The listing builds one solid part. Answer for the finished solid, in the listing's coordinates (mm). A direction names the side the tool comes from. Coordinates: 2 decimals unless noted, no trailing zeros. Write each loop counter-clockwise with the first axis right and the second up, starting at its lowest first coordinate (ties: lowest second). Pieces come first, ordered by that corner, then holes.
from build123d import *

# Parameters (mm, degrees)
SKETCH2_R                = 5
SKETCH2_R_2              = 1.5
HOLES_DEPTH              = 4
SPOKES_DEPTH             = 4
FILLET2_R                = 2
CIRPATTERN2_COUNT        = 4
FILLET2_OF_CIRPATTERN2_R = 2


with BuildPart() as part:
    # Sketch1 → Revolve1 (revolve)
    with BuildSketch(Plane.XY):
        Polygon((2, 0), (2, 39), (17, 39), (17, 44), (0, 44), (0, 0), align=None)
    revolve1 = revolve(axis=Axis((2, 0, 0), (-1, 0, 0)))

    # Mirror1: Revolve1 across plane
    add(revolve1.mirror(Plane.ZY))

    # Sketch2 → holes (cut)
    with BuildSketch(Plane(origin=(2, 0, 0), x_dir=(0, 0, -1), z_dir=(1, 0, 0))):
        with Locations(Location((0, 0, 0), (0, 0, 90))):
            Circle(SKETCH2_R)
        with Locations(Location((8, 0, 0), (0, 0, 90))):
            Circle(SKETCH2_R_2)
        with Locations(Location((0, -8, 0), (0, 0, 90))):
            Circle(SKETCH2_R_2)
        with Locations(Location((-8, 0, 0), (0, 0, 90))):
            Circle(SKETCH2_R_2)
        with Locations(Location((0, 8, 0), (0, 0, 90))):
            Circle(SKETCH2_R_2)
    extrude(amount=-HOLES_DEPTH, mode=Mode.SUBTRACT)

    # Sketch3 → spokes (cut)
    with BuildSketch(Plane(origin=(2, 0, 0), x_dir=(0, 0, -1), z_dir=(1, 0, 0))):
        with BuildLine():
            Line((8.131727984, 16.131727984), (16.131727984, 8.131727984))
            Line((16.131727984, 8.131727984), (31.131727984, 8.131727984))
            ThreePointArc((31.131727984, 8.131727984), (22.752027242, 22.752027242), (8.131727984, 31.131727984))
            Line((8.131727984, 31.131727984), (8.131727984, 16.131727984))
        make_face()
    spokes = extrude(amount=-SPOKES_DEPTH, mode=Mode.SUBTRACT)

    # Fillet2
    fillet2_edges = [part.edges().sort_by_distance(p)[0] for p in [
        (0, 16.131727984, -8.131727984),
        (0, 8.131727984, -16.131727984),
        (0, 8.131727984, -31.131727984),
        (0, 31.131727984, -8.131727984),
    ]]
    fillet(fillet2_edges, radius=FILLET2_R)

    # CirPattern2: spokes ×4 about axis
    cirpattern2_axis = Axis((0, 0, 0), (1, 0, 0))
    for i in range(1, CIRPATTERN2_COUNT):
        add(spokes.rotate(cirpattern2_axis, i * 360 / CIRPATTERN2_COUNT), mode=Mode.SUBTRACT)

    # Fillet2 of CirPattern2
    fillet2_of_cirpattern2_edges = [part.edges().sort_by_distance(p)[0] for p in [
        (0, 8.131727984, 16.131727984),
        (0, 16.131727984, 8.131727984),
        (0, 31.131727984, 8.131727984),
        (0, 8.131727984, 31.131727984),
        (0, -16.131727984, 8.131727984),
        (0, -8.131727984, 16.131727984),
        (0, -8.131727984, 31.131727984),
        (0, -31.131727984, 8.131727984),
        (0, -8.131727984, -16.131727984),
        (0, -16.131727984, -8.131727984),
        (0, -31.131727984, -8.131727984),
        (0, -8.131727984, -31.131727984),
    ]]
    fillet(fillet2_of_cirpattern2_edges, radius=FILLET2_OF_CIRPATTERN2_R)


solid = part.part
1. Flat-ended cylindrical pins translate along their axes: P1, Ø1.2, axis at x = 0, z = 20, coming from the -Y side; P2, Ø12, axis at x = -1.5, y = 4.5, coming from the -Z side; P3, Ø2, axis at x = 0, y = 24.5, coming from the +Z side. Find the tip coordinate at first contact, or state that the pin passes through.
Results found:
P1: stops at y = -39.49
P2: stops at z = -44
P3: stops at z = 37.2
2. A tool of negligible diameter and unlimited length cuts with its end or side. For faces 1 (the flat face through (-2, -8, 8)), 2 (the cylindrical face through (0.028, -22.893, -22.61)), 3 (the flat face through (2, -8, 8)), from which of +Z, -Z, +X, -X, +Y, -Y can it reach the whole face along a straight path? Write none if from no direction.
Results found:
face 1: -X
face 2: +X, -X
face 3: +X
3. Section A-A on z = 0 is taken. Give the vertices of the cut face in (x, y).
Results found:
outline: (-17, -44) - (17, -44) - (17, -39) - (2, -39) - (2, -9.5) - (-2, -9.5) - (-2, -39) - (-17, -39) - close; (-17, 39) - (-2, 39) - (-2, 9.5) - (2, 9.5) - (2, 39) - (17, 39) - (17, 44) - (-17, 44) - close; (-2, -6.5) - (2, -6.5) - (2, -5) - (-2, -5) - close; (-2, 5) - (2, 5) - (2, 6.5) - (-2, 6.5) - close
4. Section B-B on x = -3.5 is taken. Give the vertices of the cut face in (y, z).
Results found:
outline: circle Ø88 at (0, 0); hole circle Ø78 at (0, 0)
5. For a pull along Y with two mould halves and no side action, classify faces 4 (the flat face through (-17, 26.3, 29.1)), 5 (the cylindrical face through (0.03, -1.08, -4.88)), 6 (the cylindrical face through (-0.028, 8.957, 30.043)) as pulls with the +Y half, pulls with the -Y half, needs draft (parallel to the pull), parting line crosses it, or undercut.
Results found:
face 4: needs draft
face 5: undercut
face 6: undercut
6. Section C-C on y = 20.5 is taken. Give the vertices of the cut face in (x, z).
Results found:
outline: (-17, -38.93) - (17, -38.93) - (17, -33.18) - (2, -33.18) - (2, -24.8) - (-2, -24.8) - (-2, -33.18) - (-17, -33.18) - close; (-17, 33.18) - (-2, 33.18) - (-2, 24.8) - (2, 24.8) - (2, 33.18) - (17, 33.18) - (17, 38.93) - (-17, 38.93) - close; (-2, -8.13) - (2, -8.13) - (2, 8.13) - (-2, 8.13) - close
7. Find the intervals of material crossed by L1, parallel to Z at x = 0, y = 0; L2, parallel to Z at x = -14, y = 0; L3, parallel to X at y = -3, z = 17.5, in increasing order.
Results found:
L1: z = -44 to -9.5, -6.5 to -5, 5 to 6.5, 9.5 to 44
L2: z = -44 to -39, 39 to 44
L3: x = -2 to 2
8. Section D-D on z = 23 is taken. Give the vertices of the cut face in (x, y).
Results found:
outline: (-17, -37.51) - (17, -37.51) - (17, -31.5) - (2, -31.5) - (2, -22.5) - (-2, -22.5) - (-2, -31.5) - (-17, -31.5) - close; (-17, 31.5) - (-2, 31.5) - (-2, 22.5) - (2, 22.5) - (2, 31.5) - (17, 31.5) - (17, 37.51) - (-17, 37.51) - close; (-2, -8.13) - (2, -8.13) - (2, 8.13) - (-2, 8.13) - close
